Design review of the part built by this model. Coordinates are the model's own, in mm. Give positions to 0.01 mm unless a question says otherwise; leave off trailing zeros. Loops run counter-clockwise (first coordinate to the right, second up) from the corner with the lowest first, then second, coordinate; pieces in that order, holes last. Notation, with made-up numbers: (88.25, 75) -> (147.25, 75) arc R18 ccw to (147.25, 87) -> close; hole circle Ø2 at (-29.75, 1). An arc over 180 degrees is marked (long way). Answer in a Markdown table with one row per item. Add a question column.
(1) For line 1 (X direction, y = -0.1, z = 7); line 2 (Y direction, x = 45.5, z = 12.5); line 3 (X direction, y = -1.15, z = 3), list the stretches that pass through material, from the lowest coordinate up.
(2) Consider section B-B on z = 15.25. Write out the cut boundary in (x, y) (1 decimal).
(3) Consider section C-C on x = 42.5. Write out the cut boundary in (y, z), then the cut area to 3 significant figures.
(4) Consider section D-D on x = 11. Write out the cut boundary in (y, z).
(5) Consider section A-A on z = 9.75. Write out the cut boundary in (x, y).
from build123d import *

# Parameters (mm, degrees)
F1_DEPTH = 2.38125
F2_R     = 2.38125
F3_DEPTH = 25.4
F5_DEPTH = 25.4


with BuildPart() as f1:
    # F0 (on Front) → F1 (new body)
    with BuildSketch(Plane.XZ):
        with BuildLine():
            Line((60.325, 19.05), (7.9375, 19.05))
            ThreePointArc((7.9375, 19.05), (2.32484, 16.72516), (0, 11.1125))
            Line((0, 11.1125), (0, 0))
            Line((0, 0), (9.525, 0))
            Line((9.525, 0), (12.110345, 7.626242))
            ThreePointArc((12.110345, 7.626242), (13.473756, 9.517878), (15.663421, 10.319465))
            Line((15.663421, 10.319465), (60.325, 12.7))
            Line((60.325, 12.7), (60.325, 19.05))
        make_face()
    extrude(amount=F1_DEPTH)

    # F2 (on face) → F3 (cut)
    with BuildSketch(Plane.XZ.offset(2.38125)):
        with Locations((7.9375, 11.1125)):
            Circle(F2_R)
    extrude(amount=-F3_DEPTH, mode=Mode.SUBTRACT)

    # F4 (on face) → F5 (cut)
    with BuildSketch(Plane.XY.offset(19.05)):
        Polygon((60.325, 0), (45.24375, 0), (60.325, -0.79375), align=None)
        Polygon((60.325, -2.38125), (60.325, -1.5875), (45.24375, -2.38125), align=None)
    extrude(amount=-F5_DEPTH, mode=Mode.SUBTRACT)


solid = f1.part
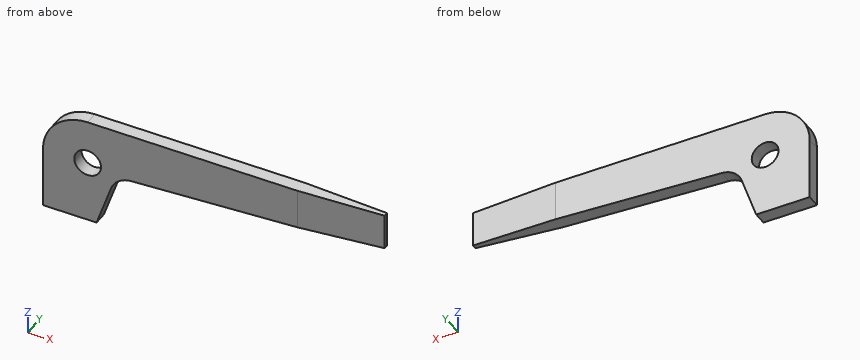
Values follow:
| question | item | result |
|---|---|---|
| 1 | line 1 | 0 to 11.9 |
| 1 | line 2 | -2.37 to -0.01 |
| 1 | line 3 | 0 to 10.54 |
| 2 | outline | (1.2, -2.4) -> (45.2, -2.4) -> (60.3, -1.6) -> (60.3, -0.8) -> (45.2, 0) -> (1.2, 0) -> close |
| 3 | outline | (-2.38, 11.75) -> (0, 11.75) -> (0, 19.05) -> (-2.38, 19.05) -> close |
| 3 | area | 17.4 mm2 |
| 4 | outline | (-2.38, 4.35) -> (0, 4.35) -> (0, 19.05) -> (-2.38, 19.05) -> close |
| 5 | outline | (0, -2.38) -> (5.98, -2.38) -> (5.98, 0) -> (0, 0) -> close; (9.89, -2.38) -> (13.82, -2.38) -> (13.82, 0) -> (9.89, 0) -> close |
